Part model, mm, in its own coordinate system. A direction names the side the tool comes from. Round coordinates to 2 decimals unless told otherwise and drop trailing zeros. Loops run counter-clockwise (first coordinate to the right, second up) from the corner with the lowest first, then second, coordinate; pieces in that order, holes last. Notation, with made-up numbers: (-39.5, 29) - (-2.5, 29) arc R18 ccw to (-2.5, 39) - close; hole circle Ø3 at (-15.75, 63.25). An arc over 180 degrees is marked (long way). Write each question's results on one line, items separated by ' | '. Start each with the question number.
(1) Cut at D-D, the plane z = 95. Give the number of separate pieces and of enclosed holes in the cut face, then the cut area to 3 significant figures.
(2) Flat gauge pins, fed straight in: P1, Ø10, axis at x = -74.5, y = 75, coming from the -Z side; P2, Ø6, axis at x = 142.5, z = 71.5, coming from the +Y side; P3, Ø8, axis at x = -47.5, z = 50.5, coming from the -Y side; P4, Ø7.5, axis at y = -148.75, z = 67.15, coming from the +X side. Where does each tip first touch, or does it go through?
(3) Drill centre lines: L1, parallel to X at y = 115, z = 174.5; L2, parallel to X at y = -101, z = 198; L3, parallel to Z at x = 275.5, y = -101.6 (3 decimals). Where is each one in solid material? Low to high.
(4) Tool access for faces 5 (the face through (1, 12, 0)), 6 (the face through (60, 25.4, 100)): list every direction of +Z, -Z, +X, -X, +Y, -Y with a clear straight run to the whole face (end or side of a thin tool).
(5) Cut at C-C, the plane y = 42.5. List the corners of the cut face in (x, z), then the cut area to 3 significant figures.
(6) Mould opens along Z. For faces 1 (the face through (-272.961, -190.472, 111.787)), 2 (the face through (2.5, 81.2, 121.8)), 3 (the face through (-272.96, -59.49, 157.58)), 4 (the face through (254, 90, 100)) say: released by +Z, released by -Z, zero draft, split by the parting line, or undercut.
(7) Cut at A-A, the plane y = -167.5. List the corners of the cut face in (x, z), then the cut area to 3 significant figures.
(8) Cut at B-B, the plane x = -195.5. List the corners of the cut face in (y, z).
from build123d import *

# Parameters (mm, degrees)
BOSS_EXTRUDE2_DEPTH = 203.2
SKETCH2_W           = 558.8
SKETCH2_H           = 25.4
BOSS_EXTRUDE3_DEPTH = 152.4
BOSS_EXTRUDE4_DEPTH = 5.08
BOSS_EXTRUDE5_DEPTH = 5.08
BOSS_EXTRUDE6_DEPTH = 5.08
SKETCH6_W           = 228.6
SKETCH6_H           = 76.2
BOSS_EXTRUDE7_DEPTH = 558.8
SKETCH7_W           = 533.4
SKETCH7_H           = 190.5
CUT_EXTRUDE1_DEPTH  = 298.590683842
SKETCH8_R           = 50.8
CUT_EXTRUDE2_DEPTH  = 634.092133895
SKETCH10_R          = 6.35
CUT_EXTRUDE3_DEPTH  = 634.092133895


with BuildPart() as part:
    # Sketch1 → Boss-Extrude2 (new body)
    with BuildSketch(Plane.XY):
        Polygon((-279.4, 0), (279.4, 0), (279.4, 152.4), (254, 152.4), (254, 25.4), (-254, 25.4), (-254, 152.4), (-279.4, 152.4), align=None)
    extrude(amount=BOSS_EXTRUDE2_DEPTH)

    # Sketch2 → Boss-Extrude3 (add)
    with BuildSketch(Plane(origin=(0, 0, 0), x_dir=(1, 0, 0), z_dir=(0, 1, 0))):
        with Locations((0, -215.9)):
            Rectangle(SKETCH2_W, SKETCH2_H)
    extrude(amount=BOSS_EXTRUDE3_DEPTH)

    # Sketch3 → Boss-Extrude4 (add)
    with BuildSketch(Plane(origin=(127, 0, 0), x_dir=(0, 0, -1), z_dir=(1, 0, 0))):
        Polygon((-228.6, 152.4), (0, 0), (-228.6, 0), align=None)
    extrude(amount=BOSS_EXTRUDE4_DEPTH)

    # Sketch4 → Boss-Extrude5 (add)
    with BuildSketch(Plane(origin=(0, 0, 0), x_dir=(0, 0, -1), z_dir=(1, 0, 0))):
        Polygon((-228.6, 152.4), (0, 0), (-228.6, 0), align=None)
    extrude(amount=BOSS_EXTRUDE5_DEPTH)

    # Sketch5 → Boss-Extrude6 (add)
    with BuildSketch(Plane(origin=(-127, 0, 0), x_dir=(0, 0, -1), z_dir=(1, 0, 0))):
        Polygon((-228.6, 152.4), (0, 0), (-228.6, 0), align=None)
    extrude(amount=-BOSS_EXTRUDE6_DEPTH)

    # Sketch6 → Boss-Extrude7 (add)
    with BuildSketch(Plane(origin=(279.4, 0, 0), x_dir=(0, 0, -1), z_dir=(1, 0, 0))):
        with Locations((-114.3, -38.1)):
            Rectangle(SKETCH6_W, SKETCH6_H)
        with BuildLine():
            Line((-228.6, -76.2), (0, -76.2))
            ThreePointArc((0, -76.2), (-114.3, -190.5), (-228.6, -76.2))
        make_face()
    extrude(amount=-BOSS_EXTRUDE7_DEPTH)

    # Sketch7 → Cut-Extrude1 (cut)
    with BuildSketch(Plane.XY):
        with Locations((0, -95.25)):
            Rectangle(SKETCH7_W, SKETCH7_H)
    extrude(amount=CUT_EXTRUDE1_DEPTH, mode=Mode.SUBTRACT)

    # Sketch8 → Cut-Extrude2 (cut, through all)
    with BuildSketch(Plane(origin=(279.4, 0, 0), x_dir=(0, 0, -1), z_dir=(1, 0, 0))):
        with Locations(Location((-114.3, -101.6, 0), (0, 0, 90))):
            Circle(SKETCH8_R)
    extrude(amount=-CUT_EXTRUDE2_DEPTH, mode=Mode.SUBTRACT)

    # Sketch10 → Cut-Extrude3 (cut, through all)
    with BuildSketch(Plane(origin=(279.4, 0, 0), x_dir=(0, 0, -1), z_dir=(1, 0, 0))):
        with Locations(Location((-114.3, -34.925, 0), (0, 0, 90))):
            Circle(SKETCH10_R)
        with Locations(Location((-67.153655364, -54.453655364, 0), (0, 0, 90))):
            Circle(SKETCH10_R)
        with Locations(Location((-47.625, -101.6, 0), (0, 0, 90))):
            Circle(SKETCH10_R)
        with Locations(Location((-67.153655364, -148.746344636, 0), (0, 0, 90))):
            Circle(SKETCH10_R)
        with Locations(Location((-114.3, -168.275, 0), (0, 0, 90))):
            Circle(SKETCH10_R)
        with Locations(Location((-161.446344636, -148.746344636, 0), (0, 0, 90))):
            Circle(SKETCH10_R)
        with Locations(Location((-180.975, -101.6, 0), (0, 0, 90))):
            Circle(SKETCH10_R)
        with Locations(Location((-161.446344636, -54.453655364, 0), (0, 0, 90))):
            Circle(SKETCH10_R)
    extrude(amount=-CUT_EXTRUDE3_DEPTH, mode=Mode.SUBTRACT)


solid = part.part
A:
1) separate pieces: 3 | enclosed holes: 0 | area: 23,600 mm2
2) P1: z = 203.2 | P2: y = 25.4 | P3: y = 0 | P4: through
3) L1: -279.4 to -254, -132.08 to -127, 0 to 5.08, 127 to 132.08, 254 to 279.4 | L2: -279.4 to -266.7, 266.7 to 279.4 | L3: 2.858 to 41.275, 53.975 to 63.5, 165.1 to 174.625, 187.325 to 225.742
4) face 5: -Z, +X, -X, +Y, -Y | face 6: -Z, +Y
5) outline: (-279.4, 0) - (-254, 0) - (-254, 203.2) - (-132.08, 203.2) - (-132.08, 63.75) - (-127, 63.75) - (-127, 203.2) - (0, 203.2) - (0, 63.75) - (5.08, 63.75) - (5.08, 203.2) - (127, 203.2) - (127, 63.75) - (132.08, 63.75) - (132.08, 203.2) - (254, 203.2) - (254, 0) - (279.4, 0) - (279.4, 228.6) - (-279.4, 228.6) - close | area: 26,600 mm2
6) face 1: split by the parting line | face 2: released by -Z | face 3: undercut | face 4: zero draft
7) outline: (-279.4, 45.53) - (-266.7, 45.53) - (-266.7, 108) - (-279.4, 108) - close; (-279.4, 120.6) - (-266.7, 120.6) - (-266.7, 183.07) - (-279.4, 183.07) - close; (266.7, 45.53) - (279.4, 45.53) - (279.4, 108) - (266.7, 108) - close; (266.7, 120.6) - (279.4, 120.6) - (279.4, 183.07) - (266.7, 183.07) - close | area: 3,170 mm2
8) outline: (0, 0) - (25.4, 0) - (25.4, 203.2) - (152.4, 203.2) - (152.4, 228.6) - (0, 228.6) - close
